Could you check a few things on this model? Use its own coordinates, in mm. A direction names the side the tool comes from. Coordinates: 2 decimals unless noted, no trailing zeros. Loops run counter-clockwise (first coordinate to the right, second up) from the corner with the lowest first, then second, coordinate; pieces in that order, holes last. Notation, with made-up numbers: (89.25, -17) - (119.25, -17) arc R20 cw to (119.25, 19) - close; hole circle Ø5 at (-2.5, -30.5). An arc over 180 degrees is marked (long way). Use CSV: the item, a comma, the result in double quotes.
from build123d import *

# Parameters (mm, degrees)
BOSS_EXTRUDE1_DEPTH = 203.2
SKETCH2_R           = 3.429
CUT_EXTRUDE1_DEPTH  = 228.981803002


with BuildPart() as part:
    # Sketch1 → Boss-Extrude1 (new body)
    with BuildSketch(Plane.XY):
        with BuildLine():
            Line((0, 0), (76.2, 0))
            Line((76.2, 0), (76.2, 6.35))
            Line((76.2, 6.35), (12.7, 6.35))
            ThreePointArc((12.7, 6.35), (8.209871939, 8.209871939), (6.35, 12.7))
            Line((6.35, 12.7), (6.35, 76.2))
            Line((6.35, 76.2), (0, 76.2))
            Line((0, 76.2), (0, 0))
        make_face()
    extrude(amount=BOSS_EXTRUDE1_DEPTH)

    # Sketch2 → Cut-Extrude1 (cut, through all)
    with BuildSketch(Plane(origin=(6.35, 0, 0), x_dir=(0, 0, -1), z_dir=(1, 0, 0))):
        with Locations(Location((-50.8, 63.5, 0), (0, 0, 90))):
            Circle(SKETCH2_R)
        with Locations(Location((-152.4, 63.5, 0), (0, 0, 90))):
            Circle(SKETCH2_R)
    extrude(amount=-CUT_EXTRUDE1_DEPTH, mode=Mode.SUBTRACT)


solid = part.part
(1) Will these pins go through, and if not, where does the flat tip stop? pin 1 (5 mm diameter, centred on x = 42.5, z = 148, fed in from +Y); pin 2 (8 mm diameter, centred on y = 63.5, z = 50.8, fed in from +X).
Computed:
pin 1,"stops at y = 6.35"
pin 2,"stops at x = 6.35"
(2) Which directions (+Z, -Z, +X, -X, +Y, -Y) give clear straight access to the entire face, cutting with the end or side of a thin tool? Please do faces 1 (the face through (6.35, 44, 100)), 2 (the face through (21, 4, 0)).
Computed:
face 1,"+Z, -Z, +X, +Y"
face 2,"-Z, +X, -X, +Y, -Y"
(3) Please list where these lines run through material, in increasing order: line 1 (Z direction, x = 5, y = 63.5); line 2 (Y direction, x = 4.5, z = 152.4); line 3 (X direction, y = 19, z = 129).
Computed:
line 1,"z = 0 to 47.37, 54.23 to 148.97, 155.83 to 203.2"
line 2,"y = 0 to 60.07, 66.93 to 76.2"
line 3,"x = 0 to 6.35"
(4) Thinking about a two-plate mould opening in Y: for faces 3 (the face through (76.2, 3, 100)), 4 (the face through (38, 0, 100)), 5 (the face through (3.22, 63.05, 155.8)), 6 (the face through (3.22, 62.76, 47.45)), which applies, +Y half, -Y half, draft (parallel to the pull), parting line (faces both ways), or undercut?
Computed:
face 3,"draft"
face 4,"-Y half"
face 5,"undercut"
face 6,"undercut"
(5) Suppose I cut it at D-D (x = 51.5). Write out the boundary of the cut face in (y, z).
Computed:
outline,"(0, 0) - (6.35, 0) - (6.35, 203.2) - (0, 203.2) - close"
(6) Suppose I cut it at A-A (z = 50.8). Write out the boundary of the cut face in (x, y).
Computed:
outline,"(0, 0) - (76.2, 0) - (76.2, 6.35) - (12.7, 6.35) arc R6.35 cw to (6.35, 12.7) - (6.35, 60.07) - (0, 60.07) - close; (0, 66.93) - (6.35, 66.93) - (6.35, 76.2) - (0, 76.2) - close"
(7) Suppose I cut it at B-B (y = 63.5). Write out the boundary of the cut face in (x, z).
Computed:
outline,"(0, 0) - (6.35, 0) - (6.35, 47.37) - (0, 47.37) - close; (0, 54.23) - (6.35, 54.23) - (6.35, 148.97) - (0, 148.97) - close; (0, 155.83) - (6.35, 155.83) - (6.35, 203.2) - (0, 203.2) - close"
(8) Suppose I cut it at C-C (z = 126). Write out the boundary of the cut face in (x, y), plus the area to 3 significant figures.
Computed:
outline,"(0, 0) - (76.2, 0) - (76.2, 6.35) - (12.7, 6.35) arc R6.35 cw to (6.35, 12.7) - (6.35, 76.2) - (0, 76.2) - close"
area,"936 mm²"
